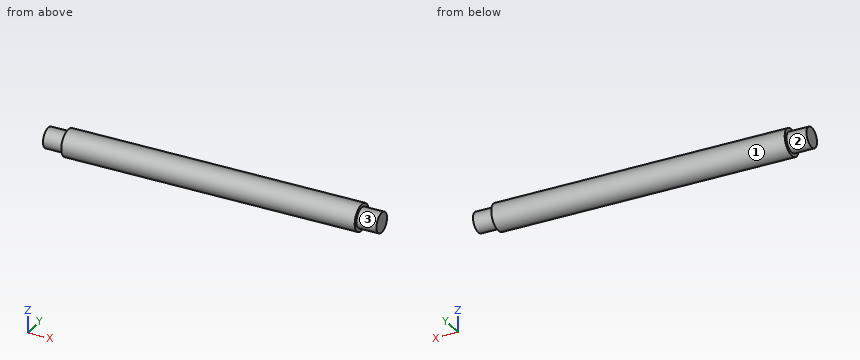
```python
from build123d import *

# Parameters (mm, degrees)
F0_R          = 7.5
F1_DEPTH      = 15
F1_DEPTH_BACK = 235
F0_R_2        = 10
F2_DEPTH      = 220


with BuildPart() as f1:
    # F0 (on Right) → F1 (new body, two sides)
    with BuildSketch(Plane.YZ) as f1_sk:
        Circle(F0_R)
    extrude(amount=F1_DEPTH)
    extrude(f1_sk.sketch, amount=-F1_DEPTH_BACK)

    # F0 (on Right) → F2 (join)
    with BuildSketch(Plane.YZ):
        Circle(F0_R_2)
        Circle(F0_R, mode=Mode.SUBTRACT)
    extrude(amount=-F2_DEPTH)


solid = f1.part
```
Here's how the part is built. I have some questions about the finished solid (model axes, mm). Face numbers are marked on the shaded views. A direction names the side the tool comes from. Give positions to 0.01 mm unless a question says otherwise; leave off trailing zeros. Order: outer loops, then holes, each group sorted by start corner. A loop starts at its lowest first (then second) coordinate and runs counter-clockwise, first axis right, second up. Notation, with made-up numbers: (-28, -33.5) - (7, -33.5) arc R14 cw to (7, -18.5) - close; hole circle Ø4 at (63, 45.25). An arc over 180 degrees is marked (long way). Answer as a JSON object with one key per item and string values. Group by question number.
Item 1: Please list where these lines run through material, in increasing order: probe 1 along X at (y, z) = (-3, -8); probe 2 along Y at (x, z) = (-22, -0.25).
Item 2: If we section it at A-A on z = 0: Please give me the cut outline in (x, y), and give its area (3 significant figures).
Item 3: For P1, Ø1, axis at x = -97, y = 3, coming from the +Z side; P2, Ø10, axis at x = -20, z = 7.5, coming from the +Y side; P3, Ø2, axis at x = -204.5, z = 8, coming from the +Y side; P4, Ø4, axis at x = -203, z = 0.5, coming from the +Y side, each with a flat end and sliding along its axis, tell me the tip position at first contact or that it passes through.
Item 4: Which directions (+Z, -Z, +X, -X, +Y, -Y) give clear straight access to the entire face, cutting with the end or side of a thin tool? Please do the marked faces 1, 2 and 3.
Item 5: If we section it at C-C on x = -142: Please give me the cut outline in (y, z).
Result set:
{
 "1": {"probe 1": "-220 to 0", "probe 2": "-10 to 10"},
 "2": {"outline": "(-235, -7.5) - (-220, -7.5) - (-220, -10) - (0, -10) - (0, -7.5) - (15, -7.5) - (15, 7.5) - (0, 7.5) - (0, 10) - (-220, 10) - (-220, 7.5) - (-235, 7.5) - close", "area": "4,850 mm²"},
 "3": {"P1": "z = 9.68", "P2": "y = 9.68", "P3": "y = 7.14", "P4": "y = 10"},
 "4": {"face 1": "+X, -X", "face 2": "-X", "face 3": "+X"},
 "5": {"outline": "circle Ø20 at (0, 0)"}
}
